Design review of the part shown in the three views and the two pictorial views. Dimensions are in mm from the part's minimum x, y and z. A direction names the side the tool comes from. Give positions to 0.01 mm unless a question says otherwise; leave off trailing zeros. Write each loop counter-clockwise with the first axis right and the second up, starting at its lowest first coordinate (ties: lowest second). Pieces come first, ordered by that corner, then holes. Notation, with made-up numbers: (2.25, 35.25) -> (24.25, 35.25) arc R13 ccw to (24.25, 45.25) -> close; hole circle Ø6 at (65.25, 76.25). An arc over 180 degrees is marked (long way). Return JSON: item names as keys, results as strings. Group by question number.
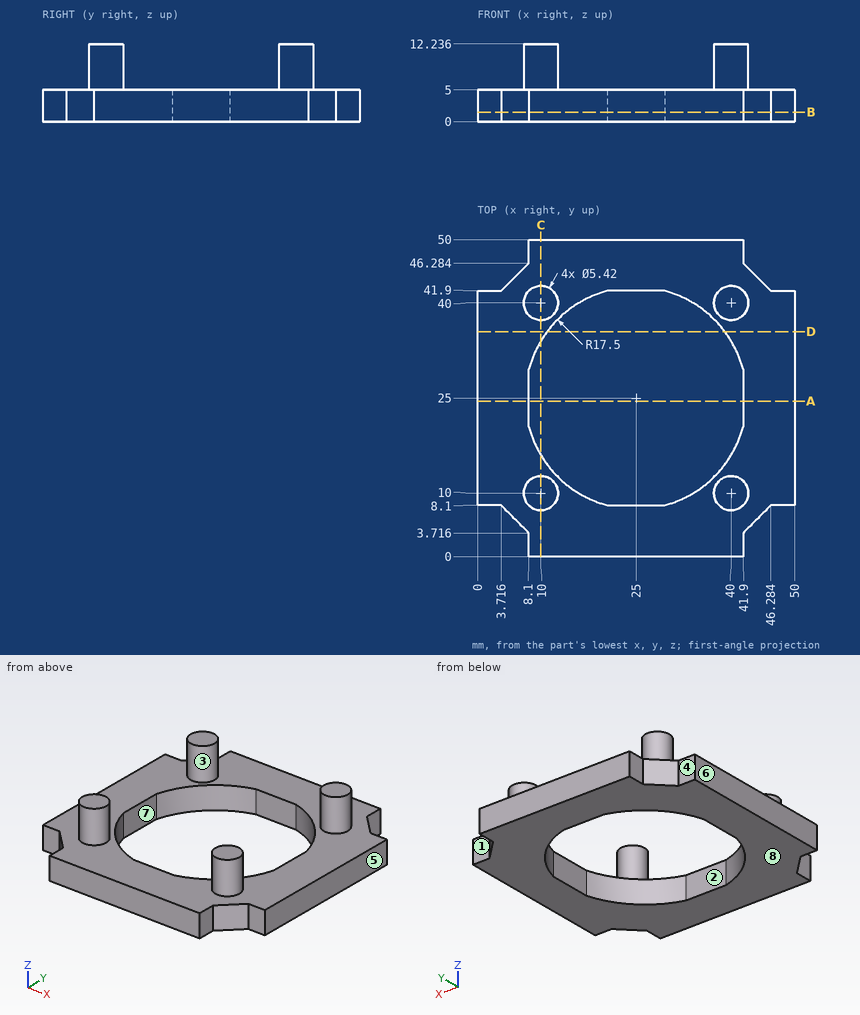
Q1. Take a section at D-D, the plane y = 35.5. Give the boundary of the cut face in (x, z).
Q2. Tool access review of the marked faces 1, 2, 3 and 4: name each direction out of +Z, -Z, +X, -X, +Y, -Y from which nothing blocks a thin tool from reaching the whole face with its end or side.
Q3. Mouldability with a two-part tool opening along X and no side actions: class the marked faces 5, 6, 7 and 8 as +X half, -X half, draft (parallel to the pull), parting line (faces both ways), or undercut.
Q4. Insertion check: pin 1 (3 mm diameter, centred on y = 48, z = 1.5, fed in from +X); pin 2 (1.1 mm diameter, centred on y = 48, z = 3, fed in from -X); pin 3 (1.1 mm diameter, centred on x = 2.5, z = 2, fed in from +Y). Each pin has a flat end and moves straight along its axis. Give the tip position at first contact, or say it passes through.
Q5. For L1, parallel to Y at x = 28, z = 3.25; L2, parallel to Z at x = 30.5, y = 4.5, list the stretches that pass through material, from the lowest coordinate up. Write a range as from..to.
Q6. Take a section at C-C, the plane x = 10. Give the boundary of the cut face in (y, z).
Q7. Take a section at B-B, the plane z = 1.5. Give the boundary of the cut face in (x, y), plus the area to 3 significant figures.
Q8. Take a section at A-A, the plane y = 24.5. Give the boundary of the cut face in (x, z), plus the area to 3 significant figures.
Final values:
{
 "1": {"outline": "(0, 0) -> (11, 0) -> (11, 5) -> (0, 5) -> close; (39, 0) -> (50, 0) -> (50, 5) -> (39, 5) -> close"},
 "2": {"face 1": "+Z, -Z, +X, +Y", "face 2": "+Z, -Z", "face 3": "+Z", "face 4": "+Z, -Z, -X, +Y"},
 "3": {"face 5": "+X half", "face 6": "-X half", "face 7": "undercut", "face 8": "draft"},
 "4": {"pin 1": "stops at x = 41.9", "pin 2": "stops at x = 8.1", "pin 3": "stops at y = 41.9"},
 "5": {"L1": "y = 0..8.1, 41.9..50", "L2": "z = 0..5"},
 "6": {"outline": "(0, 0) -> (15.99, 0) -> (15.99, 5) -> (12.71, 5) -> (12.71, 12.24) -> (7.29, 12.24) -> (7.29, 5) -> (0, 5) -> close; (34.01, 0) -> (50, 0) -> (50, 5) -> (42.71, 5) -> (42.71, 12.24) -> (37.29, 12.24) -> (37.29, 5) -> (34.01, 5) -> close"},
 "7": {"outline": "(0, 8.1) -> (3.72, 8.1) -> (8.1, 3.72) -> (8.1, 0) -> (41.9, 0) -> (41.9, 3.72) -> (46.28, 8.1) -> (50, 8.1) -> (50, 41.9) -> (46.28, 41.9) -> (41.9, 46.28) -> (41.9, 50) -> (8.1, 50) -> (8.1, 46.28) -> (3.72, 41.9) -> (0, 41.9) -> close; hole (8.1, 20.46) arc R17.5 ccw to (20.46, 8.1) -> (29.54, 8.1) arc R17.5 ccw to (41.9, 20.46) -> (41.9, 29.54) arc R17.5 ccw to (29.54, 41.9) -> (20.46, 41.9) arc R17.5 ccw to (8.1, 29.54) -> close", "area": "1,330 mm²"},
 "8": {"outline": "(0, 0) -> (8.1, 0) -> (8.1, 5) -> (0, 5) -> close; (41.9, 0) -> (50, 0) -> (50, 5) -> (41.9, 5) -> close", "area": "81.0 mm²"}
}
